Answer from the drawing. Dimensions are ordinates in mm from the lowest x, y and z of the part. A direction names the side the tool comes from. Give positions to 0.01 mm unless a question says otherwise; leave off trailing zeros. Loops run counter-clockwise (first coordinate to the right, second up) from the corner with the lowest first, then second, coordinate; pieces in that order, holes last. Notation, with made-up numbers: (-37, 86.5) - (-3, 86.5) arc R22 ccw to (-3, 105.5) - close; hole circle Ø1 at (42, 10.5). An arc over 180 degrees is marked (long way). Put each result on its own line as item: value. Start each with the question number.
1. Given pin 1 Ø5 at (x, y) = (789, 256) entering from -Z, flat-ended and moving along its own axis, determine where the tip first touches the part or whether it passes through.
2. For a pull along X with two mould halves and no side action, classify the marked faces 4, 5 and 6 as released by +X, released by -X, zero draft, split by the parting line, or undercut.
3. A cutting plane is placed at C-C, the plane y = 633. Determine the outline of the cut face in (x, z).
4. A cutting plane is placed at D-D, the plane z = 287.5. Determine the outline of the cut face in (x, y) (1 decimal).
5. For the marked faces 1, 2 and 3, determine the directions among +Z, -Z, +X, -X, +Y, -Y from which every point of the face is accessible in a straight line to the end or side of a thin tool.
6. A cutting plane is placed at B-B, the plane x = 900. Determine the outline of the cut face in (y, z), plus the area to 3 significant figures.
7. Consider L1, parallel to Y at x = 892.5, z = 103; L2, parallel to X at y = 311.5, z = 408.5; L3, parallel to X at y = 507.5, z = 183. Determine where each line is inside the solid, lowest interval first. Write a range as from..to.
8. A cutting plane is placed at A-A, the plane y = 368. Determine the outline of the cut face in (x, z), plus the area to 3 significant figures.
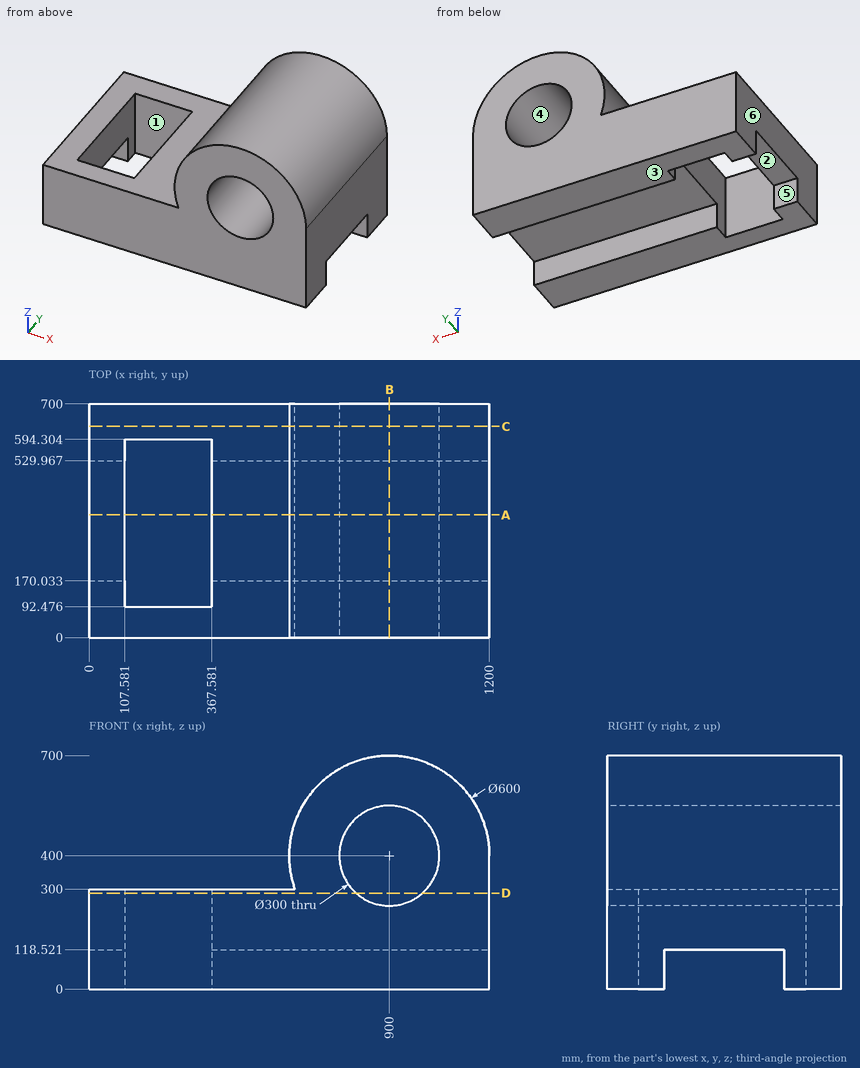
Return value:
1. pin 1: stops at z = 118.52
2. face 4: undercut
2. face 5: zero draft
2. face 6: released by -X
3. outline: (0, 0) - (1200, 0) - (1200, 400) arc R300 ccw (long way) to (617.16, 300) - (0, 300) - close; hole circle Ø300 at (900, 400)
4. outline: (0, 0) - (800.8, 0) - (800.8, 700) - (0, 700) - close; (999.2, 0) - (1200, 0) - (1200, 700) - (999.2, 700) - close; hole (107.6, 92.5) - (367.6, 92.5) - (367.6, 594.3) - (107.6, 594.3) - close
5. face 1: +Z, -Z
5. face 2: -Z, +X, -X
5. face 3: -Z, +X, -X, +Y, -Y
6. outline: (0, 0) - (170.03, 0) - (170.03, 118.52) - (529.97, 118.52) - (529.97, 0) - (700, 0) - (700, 250) - (0, 250) - close; (0, 550) - (700, 550) - (700, 700) - (0, 700) - close
6. area: 237,000 mm2
7. L1: y = 0..170.03, 529.97..700
7. L2: x = 600.12..750.24, 1049.76..1199.88
7. L3: x = 0..107.58, 367.58..1200
8. outline: (0, 118.52) - (107.58, 118.52) - (107.58, 300) - (0, 300) - close; (367.58, 118.52) - (1200, 118.52) - (1200, 400) arc R300 ccw (long way) to (617.16, 300) - (367.58, 300) - close; hole circle Ø300 at (900, 400)
8. area: 301,000 mm2
